Geometry: see drawing. Coordinates: mm, zero at the bounding-box minimum. Round coordinates to 2 decimals unless told otherwise and drop trailing zeros. Loops run counter-clockwise (first coordinate to the right, second up) from the corner with the lowest first, then second, coordinate; pieces in that order, holes last.
(1) Line query: line 1 (Y direction, x = 6, z = 1.35); line 2 (X direction, y = 6.5, z = 1.4); line 3 (X direction, y = 4.5, z = 1.2). Output: solid intervals per line, ascending.
(2) Cut plane A-A, the plane z = 1.8. Output: boundary loops of the cut face in (x, y).
(3) Draft query along Y for the marked faces 1, 2, 3 and 4. Return one class per face: released by +Y, released by -Y, zero draft, split by the parting line, or undercut.
(4) Cut plane C-C, the plane y = 11.25. Output: boundary loops of the cut face in (x, z).
(5) Cut plane B-B, the plane x = 10.5. Output: boundary loops of the cut face in (y, z), and give its area (3 significant figures).
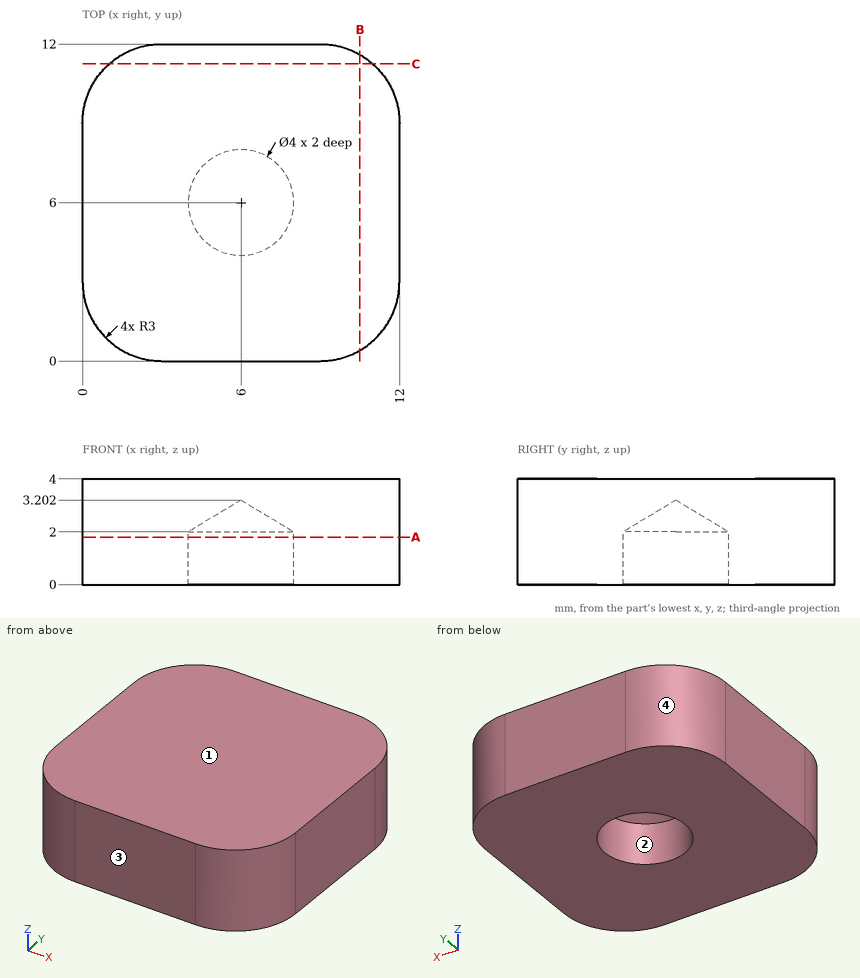
Reported:
1. line 1: y = 0 to 4, 8 to 12
1. line 2: x = 0 to 4.06, 7.94 to 12
1. line 3: x = 0 to 4.68, 7.32 to 12
2. outline: (0, 3) arc R3 ccw to (3, 0) - (9, 0) arc R3 ccw to (12, 3) - (12, 9) arc R3 ccw to (9, 12) - (3, 12) arc R3 ccw to (0, 9) - close; hole circle Ø4 at (6, 6)
3. face 1: zero draft
3. face 2: undercut
3. face 3: released by -Y
3. face 4: released by +Y
4. outline: (1.02, 0) - (10.98, 0) - (10.98, 4) - (1.02, 4) - close
5. outline: (0.4, 0) - (11.6, 0) - (11.6, 4) - (0.4, 4) - close
5. area: 44.8 mm2
